Answer from the drawing. Dimensions are ordinates in mm from the lowest x, y and z of the part. Coordinates: 2 decimals unless noted, no trailing zeros. Write each loop counter-clockwise with the first axis right and the second up, starting at its lowest first coordinate (ties: lowest second). Pieces come first, ordered by that corner, then holes.
(1) Determine the mould class of the marked faces 1, 2, 3 and 4 for opening direction Z: pulls with the +Z half, pulls with the -Z half, needs draft (parallel to the pull), parting line crosses it, or undercut.
(2) The part is cut by section D-D, the plane z = 12.25. Determine the outline of the cut face in (x, y).
(3) Given pin 1 (2.5 mm diameter, centred on y = 11.1, z = 7.5, fed in from -X); pin 2 (3 mm diameter, centred on x = 10.5, z = 8.5, fed in from +Y); pin 3 (1.5 mm diameter, centred on y = 24, z = 6.5, fed in from -X), each flat-ended and moving along its own axis, determine where each tip first touches the part or whether it passes through.
(4) Straight lines are drawn through the part: line 1 along X through (y, z) = (6, 13); line 2 along Y through (x, z) = (7.5, 10.75). For each, find the intervals that lie inside material, in ascending order.
(5) The part is cut by section A-A, the plane z = 7.5. Determine the outline of the cut face in (x, y).
(6) The part is cut by section B-B, the plane x = 7.5. Determine the outline of the cut face in (y, z).
(7) The part is cut by section C-C, the plane y = 10.5. Determine the outline of the cut face in (x, z).
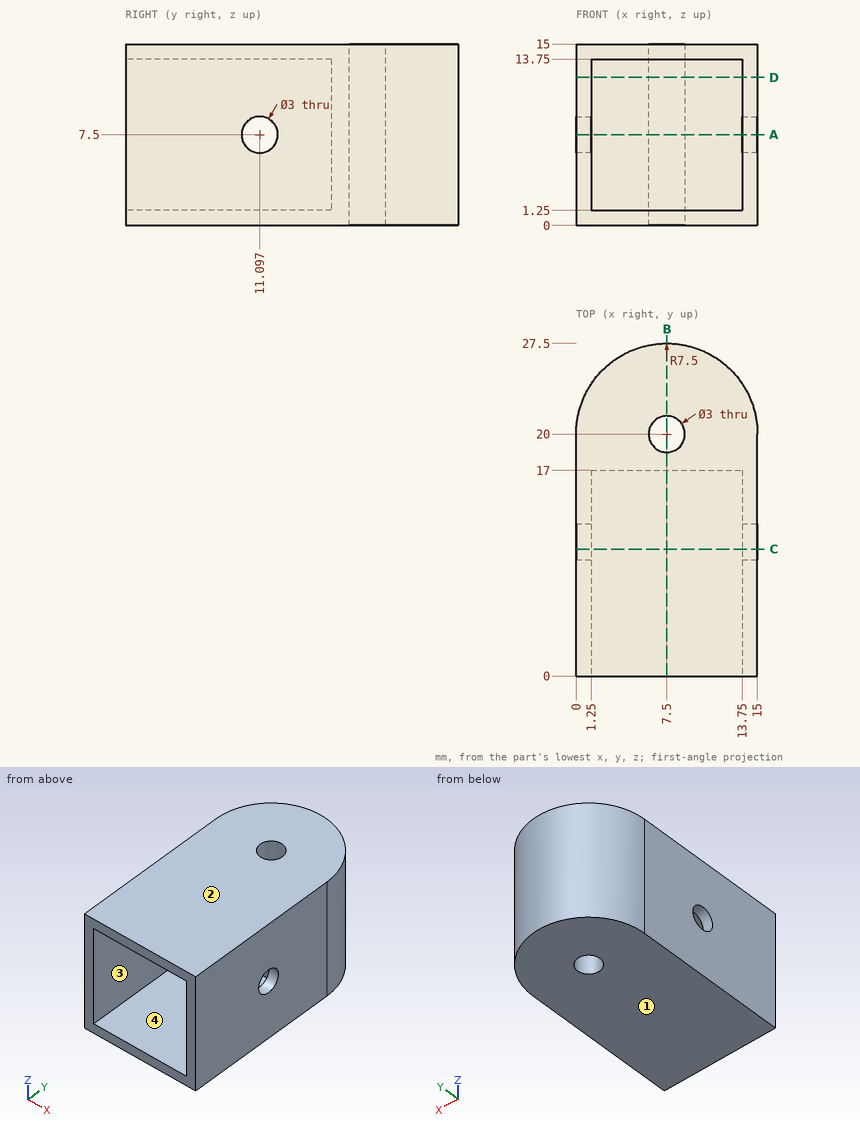
Computed:
1. face 1: pulls with the -Z half
1. face 2: pulls with the +Z half
1. face 3: undercut
1. face 4: undercut
2. outline: (0, 0) - (1.25, 0) - (1.25, 17) - (13.75, 17) - (13.75, 0) - (15, 0) - (15, 20) arc R7.5 ccw to (0, 20) - close; hole circle Ø3 at (7.5, 20)
3. pin 1: passes through
3. pin 2: stops at y = 27.35
3. pin 3: stops at x = 0.74
4. line 1: x = 0 to 1.25, 13.75 to 15
4. line 2: y = 17 to 18.5, 21.5 to 27.5
5. outline: (0, 0) - (1.25, 0) - (1.25, 9.6) - (0, 9.6) - close; (0, 12.6) - (1.25, 12.6) - (1.25, 17) - (13.75, 17) - (13.75, 12.6) - (15, 12.6) - (15, 20) arc R7.5 ccw to (0, 20) - close; (13.75, 0) - (15, 0) - (15, 9.6) - (13.75, 9.6) - close; hole circle Ø3 at (7.5, 20)
6. outline: (0, 0) - (18.5, 0) - (18.5, 15) - (0, 15) - (0, 13.75) - (17, 13.75) - (17, 1.25) - (0, 1.25) - close; (21.5, 0) - (27.5, 0) - (27.5, 15) - (21.5, 15) - close
7. outline: (0, 0) - (15, 0) - (15, 6.12) - (13.75, 6.12) - (13.75, 1.25) - (1.25, 1.25) - (1.25, 6.12) - (0, 6.12) - close; (0, 8.88) - (1.25, 8.88) - (1.25, 13.75) - (13.75, 13.75) - (13.75, 8.88) - (15, 8.88) - (15, 15) - (0, 15) - close
